Geometry check sheet. Reference: the model listing, model coordinates, mm. Face numbers are marked on the shaded views. A direction names the side the tool comes from. Coordinates: 2 decimals unless noted, no trailing zeros. Loops run counter-clockwise (first coordinate to the right, second up) from the corner with the lowest first, then second, coordinate; pieces in that order, holes last.
from build123d import *

# Parameters (mm, degrees)
F0_W        = 38.1
F0_H        = 22.86
F1_DEPTH    = 33.02
F4_DEPTH    = 25.4
F5_T1_DEPTH = 128.3541230591


# Not quite as in the source:
# - a fillet or chamfer that OpenCascade refuses, or shapes differently, is made with other operations: its cross-section is extruded or revolved along the edge and cut away or added


with BuildPart() as f1:
    # F0 (on Top) → F1 (new body)
    with BuildSketch(Plane.XY):
        with Locations((19.05, -11.43)):
            Rectangle(F0_W, F0_H)
    extrude(amount=F1_DEPTH)

    # F3 (on face) → F4 (cut)
    with BuildSketch(Plane.XZ.offset(22.86)):
        with BuildLine():
            Line((0, 22.3022773862), (0, 0))
            Line((0, 0), (38.1, 0))
            Line((38.1, 0), (38.1, 16.51))
            add(Edge.make_bspline(
                [(0, 22.3022773862), (4.0173555015, 15.4189654394), (12.5954888388, 0.7212450957), (28.7387394496, 12.7226787633), (38.1, 16.51)],
                knots=[0, 0, 0, 0, 0.2888963968, 0.6168714248, 0.6168714248, 0.6168714248, 0.6168714248], degree=3))
        make_face()
        Polygon((0, 33.02), (0, 27.94), (15.24, 27.94), (15.24, 20.32), (38.1, 20.32), (38.1, 33.02), align=None)
    extrude(amount=-F4_DEPTH, mode=Mode.SUBTRACT)

    # F5: fillet of radius 33.02 on 1 edges, made by hand

    # F5_s2 → F5_t1 (cut)
    with BuildSketch(Plane.XZ.offset(-52.7470615295)):
        with BuildLine():
            ThreePointArc((-5.8588246118, 27.94), (5.3575116884, 25.976628922), (15.24, 20.32))
            Line((15.24, 20.32), (15.24, 27.94))
            Line((15.24, 27.94), (-5.8588246118, 27.94))
        make_face()
    extrude(amount=F5_T1_DEPTH, mode=Mode.SUBTRACT)


solid = f1.part
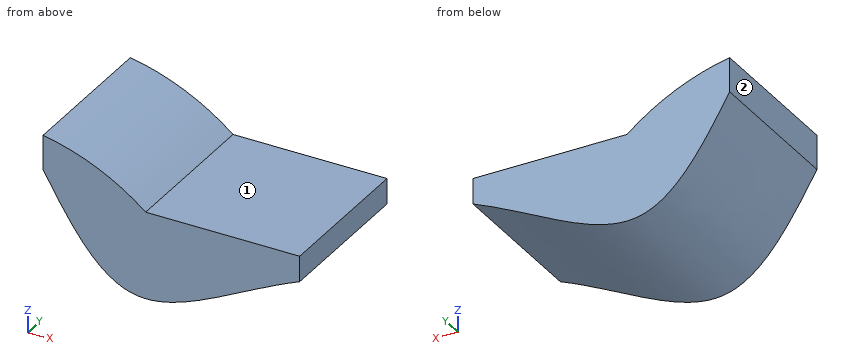
1) Material ranges on probe 1 along Z at (x, y) = (2, -13.25); probe 2 along Z at (x, y) = (16.5, -20.25); probe 3 along X at (y, z) = (-10, 18.25), recorded low to high.
Data:
probe 1: z = 18.91 to 26.99
probe 2: z = 7.43 to 20.32
probe 3: x = 2.4 to 38.1
2) Depth check by flat-ended pin: pin 1 (2 mm diameter, centred on x = 26.5, y = -15.5, fed in from +Z); pin 2 (1 mm diameter, centred on y = -20, z = 11.5, fed in from -X); pin 3 (4 mm diameter, centred on y = -15.5, z = 9.5, fed in from -X). Enter the tip coordinate at first touch or a pass-through.
Data:
pin 1: stops at z = 20.32
pin 2: stops at x = 6.83
pin 3: stops at x = 7.28
3) Access from +Z, -Z, +X, -X, +Y, -Y to the whole of each face (thin tool, end or side, straight path). Record for the marked faces 1 and 2.
Data:
face 1: +Z, +X, +Y, -Y
face 2: +Z, -Z, -X, +Y, -Y
4) Section check A-A on z = 24. Record the cut outline in (x, y), and give its area (3 significant figures).
Data:
outline: (0, -22.86) - (9.78, -22.86) - (9.78, 0) - (0, 0) - close
area: 224 mm2
